from build123d import *

# Parameters (mm, degrees)
SKETCH_1_W           = 4.2
SKETCH_1_H           = 3.2
EXTRUDE_1_DEPTH      = 5
SKETCH_2_W           = 3.6
SKETCH_2_H           = 2.6
CUT_EXTRUDE_2_DEPTH  = 4.5
SKETCH_10_W          = 1.719860591
SKETCH_10_H          = 0.3
CUT_EXTRUDE_6_DEPTH  = 1.5
EXTRUDE_2_DEPTH      = 4
EXTRUDE_2_DEPTH_BACK = 2
SKETCH_12_W          = 0.497980778
SKETCH_12_H          = 0.499968878
SKETCH_12_W_2        = 0.49954636
CHAMFER_2_SIZE       = 0.1
CHAMFER_3_SIZE       = 0.1
SKETCH_13_W          = 0.786936725
SKETCH_13_H          = 0.841611244
CUT_EXTRUDE_7_DEPTH  = 0.5


with BuildPart() as part:
    # 草图1 → 凸台-拉伸1 (new body)
    with BuildSketch(Plane.XY):
        Rectangle(SKETCH_1_W, SKETCH_1_H)
    extrude(amount=EXTRUDE_1_DEPTH)

    # 草图2 → 切除-拉伸2 (cut)
    with BuildSketch(Plane.XY.offset(5)):
        Rectangle(SKETCH_2_W, SKETCH_2_H)
    extrude(amount=-CUT_EXTRUDE_2_DEPTH, mode=Mode.SUBTRACT)

    # 草图10 → 切除-拉伸6 (cut)
    with BuildSketch(Plane.XY.offset(5)):
        with Locations((-0.021149262, 1.45)):
            Rectangle(SKETCH_10_W, SKETCH_10_H)
    extrude(amount=-CUT_EXTRUDE_6_DEPTH, mode=Mode.SUBTRACT)

    # 草图12 → 凸台-拉伸2 (add, two sides: drawn at the far end of the back side and taken through both)
    with BuildSketch(Plane.XY.offset(0.5).offset(-EXTRUDE_2_DEPTH_BACK)):
        with Locations((-0.7, -0.4)):
            Rectangle(SKETCH_12_W, SKETCH_12_H)
        with Locations((0.7, -0.4)):
            Rectangle(SKETCH_12_W_2, SKETCH_12_H)
    extrude(amount=EXTRUDE_2_DEPTH + EXTRUDE_2_DEPTH_BACK)

    # 倒角2
    chamfer_2_edges = [part.edges().sort_by_distance(p)[0] for p in [
        (-0.451009611, -0.4, 4.5),
        (-0.7, -0.150015561, 4.5),
        (-0.948990389, -0.4, 4.5),
        (-0.7, -0.649984439, 4.5),
        (0.94977318, -0.4, 4.5),
        (0.7, -0.150015561, 4.5),
        (0.45022682, -0.4, 4.5),
        (0.7, -0.649984439, 4.5),
    ]]
    chamfer(chamfer_2_edges, length=CHAMFER_2_SIZE)

    # 倒角3
    chamfer_3_edges = [part.edges().sort_by_distance(p)[0] for p in [
        (-0.451009611, -0.4, -1.5),
        (-0.7, -0.649984439, -1.5),
        (-0.948990389, -0.4, -1.5),
        (-0.7, -0.150015561, -1.5),
        (0.94977318, -0.4, -1.5),
        (0.7, -0.649984439, -1.5),
        (0.45022682, -0.4, -1.5),
        (0.7, -0.150015561, -1.5),
    ]]
    chamfer(chamfer_3_edges, length=CHAMFER_3_SIZE)

    # 草图13 → 切除-拉伸7 (cut)
    with BuildSketch(Plane.XZ.offset(1.6)):
        with Locations((-0.221312495, 3.247007401)):
            Rectangle(SKETCH_13_W, SKETCH_13_H)
    extrude(amount=-CUT_EXTRUDE_7_DEPTH, mode=Mode.SUBTRACT)


solid = part.part
Input: part model. Units: mm. Frame: model coordinates. A direction names the side the tool comes from. Coordinates: 2 decimals unless noted, no trailing zeros. Loops run counter-clockwise (first coordinate to the right, second up) from the corner with the lowest first, then second, coordinate; pieces in that order, holes last.
(1) Material intervals for probe 1 along X at (y, z) = (-0.25, 0.75); probe 2 along Y at (x, z) = (1.75, 0.75); probe 3 along X at (y, z) = (1.25, 2), sorted ascending.
(2) Section C-C on x = 1.65. Return the cut outline in (y, z), then the cut area to 3 significant figures.
(3) Section B-B on z = 1.75. Return the cut outline in (x, y), then the cut area to 3 significant figures.
(4) Set-up query: faces 4 (the face through (0.4, -1.3, 2.8)), 5 (the face through (-2.1, 0, 2)). Return all of +Z, -Z, +X, -X, +Y, -Y with unobstructed straight access to the full face (end or side cutting, diameter ignored); none if empty.
(5) Section D-D on x = -0.2. Return the cut outline in (y, z).
(6) First-contact query: pin 1 Ø0.5 at (y, z) = (-0.5, -0.5) entering from +X. Flat tip, straight axial feed; report the tip coordinate or a pass-through.
(7) Pull-direction query (Y, two-part tool) for faces 1 (the face through (0, -1.6, 2)), 2 (the face through (0, 0, 0)), 3 (the face through (1.8, 0, 3)); classes: released by +Y, released by -Y, zero draft, split by the parting line, or undercut.
(8) Section A-A on z = -0.25. Return the cut outline in (x, y).
Data:
1. probe 1: x = -2.1 to -1.8, -0.95 to -0.45, 0.45 to 0.95, 1.8 to 2.1
1. probe 2: y = -1.6 to -1.3, 1.3 to 1.6
1. probe 3: x = -2.1 to -1.8, 1.8 to 2.1
2. outline: (-1.6, 0) - (1.6, 0) - (1.6, 5) - (1.3, 5) - (1.3, 0.5) - (-1.3, 0.5) - (-1.3, 5) - (-1.6, 5) - close
2. area: 4.30 mm2
3. outline: (-2.1, -1.6) - (2.1, -1.6) - (2.1, 1.6) - (-2.1, 1.6) - close; (-0.95, -0.65) - (-0.45, -0.65) - (-0.45, -0.15) - (-0.95, -0.15) - close; (0.45, -0.65) - (0.95, -0.65) - (0.95, -0.15) - (0.45, -0.15) - close; hole (-1.8, -1.3) - (1.8, -1.3) - (1.8, 1.3) - (-1.8, 1.3) - close
3. area: 4.58 mm2
4. face 4: +Z
4. face 5: +Z, -Z, -X, +Y, -Y
5. outline: (-1.6, 0) - (1.6, 0) - (1.6, 3.5) - (1.3, 3.5) - (1.3, 0.5) - (-1.3, 0.5) - (-1.3, 2.83) - (-1.6, 2.83) - close; (-1.6, 3.67) - (-1.3, 3.67) - (-1.3, 5) - (-1.6, 5) - close
6. pin 1: stops at x = 0.95
7. face 1: released by -Y
7. face 2: zero draft
7. face 3: undercut
8. outline: (-0.95, -0.65) - (-0.45, -0.65) - (-0.45, -0.15) - (-0.95, -0.15) - close; (0.45, -0.65) - (0.95, -0.65) - (0.95, -0.15) - (0.45, -0.15) - close
